Part model, mm, in its own coordinate system. A direction names the side the tool comes from. Coordinates: 2 decimals unless noted, no trailing zeros. Write each loop counter-clockwise with the first axis right and the second up, starting at its lowest first coordinate (ties: lowest second). Pieces come first, ordered by that corner, then holes. Notation, with made-up numbers: (-18.5, 51.5) - (8.5, 51.5) arc R17 ccw to (8.5, 71.5) - close; hole circle Ø2 at (-21, 17.5). An arc over 180 degrees is marked (long way). Write each question's results on one line, items separated by ' | '.
from build123d import *

# Parameters (mm, degrees)
SKETCH1_W           = 54.5
SKETCH1_H           = 34.5
BOSS_EXTRUDE1_DEPTH = 1
SKETCH6_W           = 5
SKETCH6_H           = 14.5
CUT_EXTRUDE1_DEPTH  = 2
SKETCH9_W           = 5
SKETCH9_H           = 14.5
CUT_EXTRUDE2_DEPTH  = 2
SKETCH27_W          = 1.5
SKETCH27_H          = 10
CUT_EXTRUDE3_DEPTH  = 2
SKETCH37_W          = 1.5
SKETCH37_H          = 10
CUT_EXTRUDE10_DEPTH = 2


with BuildPart() as part:
    # Sketch1 → Boss-Extrude1 (new body)
    with BuildSketch(Plane(origin=(0, 0, 0), x_dir=(1, 0, 0), z_dir=(0, 1, 0))):
        Rectangle(SKETCH1_W, SKETCH1_H)
    extrude(amount=BOSS_EXTRUDE1_DEPTH)

    # Sketch6 → Cut-Extrude1 (cut)
    with BuildSketch(Plane(origin=(0, 1, 0), x_dir=(1, 0, 0), z_dir=(0, 1, 0))):
        with Locations((-12.75, 6)):
            Rectangle(SKETCH6_W, SKETCH6_H)
    extrude(amount=-CUT_EXTRUDE1_DEPTH, mode=Mode.SUBTRACT)

    # Sketch9 → Cut-Extrude2 (cut)
    with BuildSketch(Plane(origin=(0, 1, 0), x_dir=(1, 0, 0), z_dir=(0, 1, 0))):
        with Locations((12.75, 6)):
            Rectangle(SKETCH9_W, SKETCH9_H)
    extrude(amount=-CUT_EXTRUDE2_DEPTH, mode=Mode.SUBTRACT)

    # Sketch27 → Cut-Extrude3 (cut)
    with BuildSketch(Plane(origin=(0, 1, 0), x_dir=(1, 0, 0), z_dir=(0, 1, 0))):
        with Locations((-21, -12.25)):
            Rectangle(SKETCH27_W, SKETCH27_H)
    extrude(amount=-CUT_EXTRUDE3_DEPTH, mode=Mode.SUBTRACT)

    # Sketch37 → Cut-Extrude10 (cut)
    with BuildSketch(Plane(origin=(0, 1, 0), x_dir=(1, 0, 0), z_dir=(0, 1, 0))):
        with Locations((3.5, -12.25)):
            Rectangle(SKETCH37_W, SKETCH37_H)
    extrude(amount=-CUT_EXTRUDE10_DEPTH, mode=Mode.SUBTRACT)


solid = part.part
(1) Saw through at B-B on x = 13. Write the cut outline in (y, z), then the cut area to 3 significant figures.
Return value:
outline: (0, -17.25) - (1, -17.25) - (1, -13.25) - (0, -13.25) - close; (0, 1.25) - (1, 1.25) - (1, 17.25) - (0, 17.25) - close | area: 20.0 mm^2
(2) 3-axis set-ups, long thin cutter, end or side, ignore diameter. For faces 5 (the flat face through (0, 1, 0)), 6 (the flat face through (4.25, 0.5, 12.3)), 7 (the flat face through (12.7, 0.5, -13.25)): which of +Z, -Z, +X, -X, +Y, -Y reach the whole face in a straight line?
Return value:
face 5: +Z, -Z, +X, -X, +Y | face 6: +Z, +Y, -Y | face 7: +Y, -Y
(3) Wall check: line 1 (X direction, y = 0.45, z = 13); line 2 (X direction, y = 0.35, z = 0); line 3 (Z direction, x = 12, y = 0.95). Give the ranges that are in metal, low to high. Write a range as from..to.
Return value:
line 1: x = -27.25..-21.75, -20.25..2.75, 4.25..27.25 | line 2: x = -27.25..-15.25, -10.25..10.25, 15.25..27.25 | line 3: z = -17.25..-13.25, 1.25..17.25
(4) Saw through at D-D on z = 9. Write the cut outline in (x, y), then the cut area to 3 significant figures.
Return value:
outline: (-27.25, 0) - (-21.75, 0) - (-21.75, 1) - (-27.25, 1) - close; (-20.25, 0) - (2.75, 0) - (2.75, 1) - (-20.25, 1) - close; (4.25, 0) - (27.25, 0) - (27.25, 1) - (4.25, 1) - close | area: 51.5 mm^2
(5) Two-plate mould, pull along Z, no slides. Class faces 1 (the flat face through (-8.9, 0.5, 17.25)), 2 (the flat face through (10.25, 0.5, -5.9)), 3 (the flat face through (0, 0, 0)), 4 (the flat face through (-10.25, 0.5, -5.9)): released by +Z, released by -Z, zero draft, split by the parting line, or undercut.
Return value:
face 1: released by +Z | face 2: undercut | face 3: zero draft | face 4: undercut
(6) Saw through at A-A on z = 0. Write the cut outline in (x, y).
Return value:
outline: (-27.25, 0) - (-15.25, 0) - (-15.25, 1) - (-27.25, 1) - close; (-10.25, 0) - (10.25, 0) - (10.25, 1) - (-10.25, 1) - close; (15.25, 0) - (27.25, 0) - (27.25, 1) - (15.25, 1) - close
(7) Saw through at C-C on y = 0.6. Write the cut outline in (x, z).
Return value:
outline: (-27.25, -17.25) - (27.25, -17.25) - (27.25, 17.25) - (4.25, 17.25) - (4.25, 7.25) - (2.75, 7.25) - (2.75, 17.25) - (-20.25, 17.25) - (-20.25, 7.25) - (-21.75, 7.25) - (-21.75, 17.25) - (-27.25, 17.25) - close; hole (-15.25, -13.25) - (-10.25, -13.25) - (-10.25, 1.25) - (-15.25, 1.25) - close; hole (10.25, -13.25) - (15.25, -13.25) - (15.25, 1.25) - (10.25, 1.25) - close
